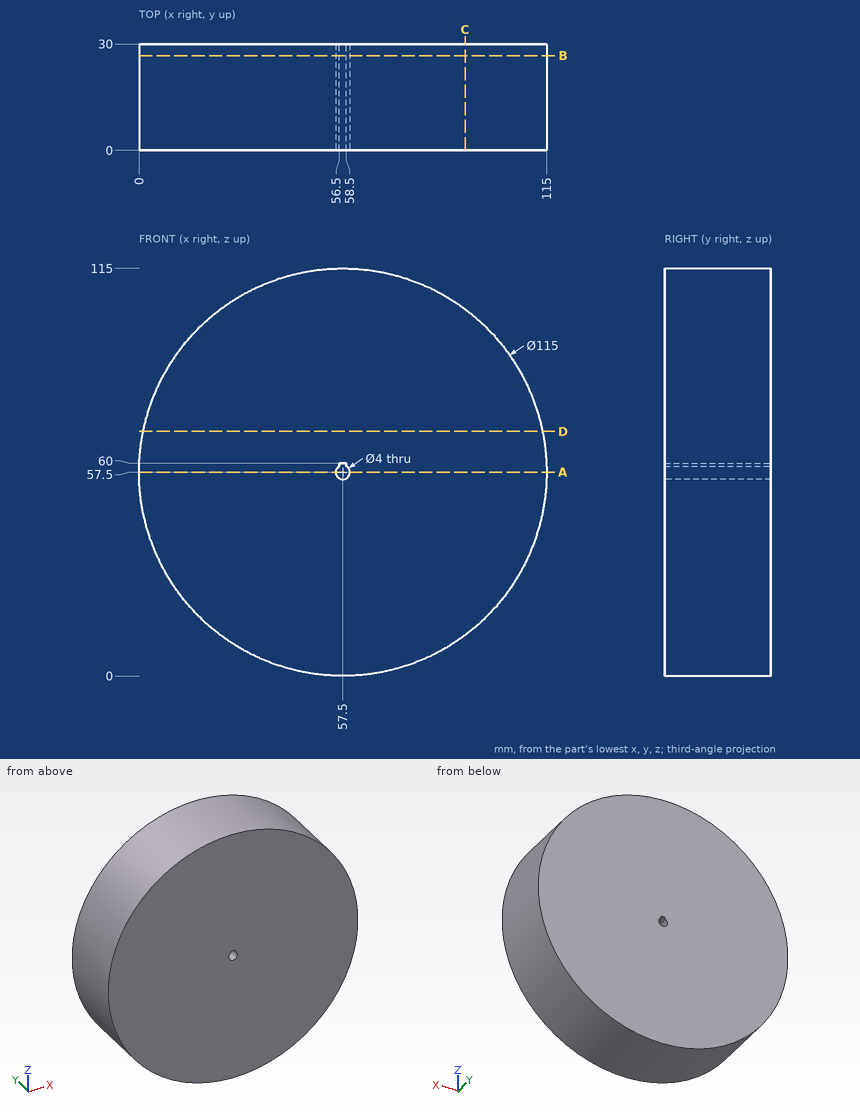
Drawing for the job (mm, zero at the part's lowest x, y, z). Give positions to 0.01 mm unless a question says otherwise; leave off trailing zeros. Order: outer loops, then holes, each group sorted by start corner. A loop starts at its lowest first (then second) coordinate and runs counter-clockwise, first axis right, second up. Notation, with made-up numbers: (13.25, 31.25) - (51.25, 31.25) arc R20 cw to (51.25, 36.25) - close; hole circle Ø9 at (49.25, -32). An arc over 180 degrees is marked (long way). Write item = value, one per line. Start each with the question number.
1. Cut at D-D, the plane z = 69. List the corners of the cut face in (x, y).
2. Cut at A-A, the plane z = 57.5. List the corners of the cut face in (x, y), and give its area (3 significant figures).
3. Drop flat-ended pins along their axis: P1, Ø1.5, axis at x = 58, y = 26, coming from the +Z side; P2, Ø10, axis at y = 20.5, z = 42, coming from the +X side; P3, Ø5, axis at y = 15.5, z = 79.5, coming from the -X side; P4, Ø12, axis at x = 40, y = 9.5, coming from the +Z side. Give the stop position or say it passes through.
4. Cut at B-B, the plane y = 26.75. List the corners of the cut face in (x, z), and give its area (3 significant figures).
5. Probe line 1 along X through (y, z) = (21, 50); line 2 along Z through (x, y) = (70.5, 6); line 3 along X through (y, z) = (5.25, 67.5). List the from-to ranges inside material, lowest first.
6. Cut at C-C, the plane x = 92. List the corners of the cut face in (y, z).
Taken from the geometry:
q1.outline = (1.16, 0) - (113.84, 0) - (113.84, 30) - (1.16, 30) - close
q2.outline = (0, 0) - (55.5, 0) - (55.5, 30) - (0, 30) - close; (59.5, 0) - (115, 0) - (115, 30) - (59.5, 30) - close
q2.area = 3,330 mm²
q3.P1 = 115
q3.P2 = 114.03
q3.P3 = 3.41
q3.P4 = 113.84
q4.outline = circle Ø115 at (57.5, 57.5); hole (56.5, 59.23) arc R2 ccw (long way) to (58.5, 59.23) - (58.5, 60) - (56.5, 60) - close
q4.area = 10,400 mm²
q5.line_1 = 0.49 to 114.51
q5.line_2 = 1.49 to 113.51
q5.line_3 = 0.88 to 114.12
q6.outline = (0, 11.5) - (30, 11.5) - (30, 103.5) - (0, 103.5) - close
